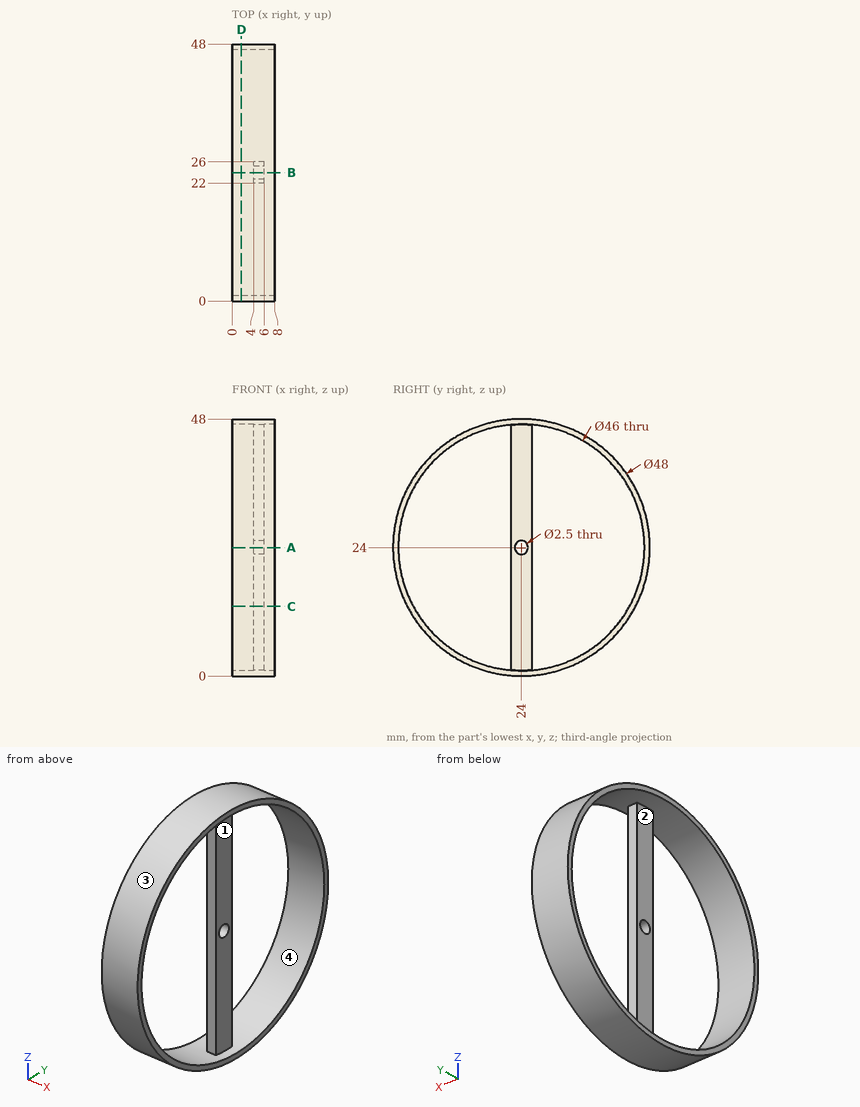
Geometry check sheet. Reference: drawing and pictorial views, mm from the part's lowest x, y, z. A direction names the side the tool comes from. Round coordinates to 2 decimals unless told otherwise and drop trailing zeros. Loops run counter-clockwise (first coordinate to the right, second up) from the corner with the lowest first, then second, coordinate; pieces in that order, holes last.
1. Sectioned sample at B-B on y = 24. Record the boundary of the cut face in (x, z), and give its area (3 significant figures).
2. Sectioned sample at C-C on z = 13. Record the boundary of the cut face in (x, y), and give its area (3 significant figures).
3. Scan lines: probe 1 along Z at (x, y) = (5, 24); probe 2 along Y at (x, z) = (5.75, 10); probe 3 along Y at (x, z) = (4.25, 17.5). Record each from-to range of solid material in increasing order.
4. Gauge pin test, flat ends, axial feed: pin 1 Ø0.6 at (x, z) = (5, 26.5) entering from -Y; pin 2 Ø0.6 at (x, z) = (5, 16.5) entering from +Y; pin 3 Ø2 at (x, z) = (6, 16) entering from +Y. Record the tip position at first contact, or that the pin passes through.
5. Sectioned sample at A-A on z = 24. Record the boundary of the cut face in (x, y).
6. Sectioned sample at D-D on x = 1.75. Record the boundary of the cut face in (y, z).
7. Mould release check, pull along Y, two halves, no side actions. Record for the marked faces 3 and 4: released by +Y, released by -Y, zero draft, split by the parting line, or undercut.
8. Set-up check for the marked faces 1 and 2: record each of +Z, -Z, +X, -X, +Y, -Y from which the full face is reachable in a straight line by a thin tool's end or side.
Recorded:
1. outline: (0, 0) - (8, 0) - (8, 1) - (6, 1) - (6, 22.75) - (4, 22.75) - (4, 1) - (0, 1) - close; (0, 47) - (4, 47) - (4, 25.25) - (6, 25.25) - (6, 47) - (8, 47) - (8, 48) - (0, 48) - close
1. area: 103 mm2
2. outline: (0, 2.67) - (8, 2.67) - (8, 3.8) - (0, 3.8) - close; (0, 44.2) - (8, 44.2) - (8, 45.33) - (0, 45.33) - close; (4, 22) - (6, 22) - (6, 26) - (4, 26) - close
2. area: 26.1 mm2
3. probe 1: z = 0 to 22.75, 25.25 to 48
3. probe 2: y = 4.51 to 5.75, 22 to 26, 42.25 to 43.49
3. probe 3: y = 0.9 to 1.94, 22 to 26, 46.06 to 47.1
4. pin 1: stops at y = 0.1
4. pin 2: stops at y = 46.89
4. pin 3: stops at y = 46.96
5. outline: (0, 0) - (8, 0) - (8, 1) - (0, 1) - close; (0, 47) - (8, 47) - (8, 48) - (0, 48) - close; (4, 22) - (6, 22) - (6, 22.75) - (4, 22.75) - close; (4, 25.25) - (6, 25.25) - (6, 26) - (4, 26) - close
6. outline: circle Ø48 at (24, 24); hole circle Ø46 at (24, 24)
7. face 3: split by the parting line
7. face 4: undercut
8. face 1: +X
8. face 2: -X
